from build123d import *

# Parameters (mm, degrees)
F0_R      = 15
F2_R      = 12.5
F4_R      = 10
F6_R      = 7.5
F8_R      = 5
F10_W     = 35
F10_H     = 35
F11_DEPTH = 1


with BuildPart() as f9:
    # F0 (on Top) → F9 section 0
    with BuildSketch(Plane.XY):
        Circle(F0_R)
    # F2 (on offset) → F9 section 1
    with BuildSketch(Plane.XY.offset(10)):
        Circle(F2_R)
    # F4 (on offset) → F9 section 2
    with BuildSketch(Plane.XY.offset(20)):
        Circle(F4_R)
    # F6 (on offset) → F9 section 3
    with BuildSketch(Plane.XY.offset(30)):
        Circle(F6_R)
    # F8 (on offset) → F9 section 4
    with BuildSketch(Plane.XY.offset(40)):
        Circle(F8_R)
    loft()

    # F10 (on Top) → F11 (join)
    with BuildSketch(Plane.XY):
        Rectangle(F10_W, F10_H)
    extrude(amount=-F11_DEPTH)


solid = f9.part
Verification items for the finished model (mm, model axes). A direction names the side the tool comes from. Give positions to 0.01 mm unless a question says otherwise; leave off trailing zeros. Answer as CSV lines item,"result". Start each with the question number.
1. Depth check by flat-ended pin: pin 1 (8 mm diameter, centred on x = -12.5, z = 9, fed in from -Y); pin 2 (5 mm diameter, centred on x = 12.5, z = 5.5, fed in from +Y); pin 3 (6 mm diameter, centred on x = 7.5, z = 7, fed in from -Y); pin 4 (1.5 mm diameter, centred on x = 9, z = 27.5, fed in from +Y). Enter the tip coordinate at first touch or a pass-through.
2. Thickness scan on line 1 (Z direction, x = 15, y = -5); line 2 (X direction, y = 10.5, z = 5.5); line 3 (Y direction, x = -9, z = 18). Record the ranges inside material, lowest first.
3. Set-up check for faces 1 (the face through (-13, -9, 0)), 2 (the face through (-0.2, -17.5, -0.5)): record each of +Z, -Z, +X, -X, +Y, -Y from which the full face is reachable in a straight line by a thin tool's end or side.
Derived:
1,pin 1,"y = -9.75"
1,pin 2,"y = 9.41"
1,pin 3,"y = -12.72"
1,pin 4,"through"
2,line 1,"-1 to 0"
2,line 2,"-8.68 to 8.68"
2,line 3,"-5.41 to 5.41"
3,face 1,"+Z"
3,face 2,"+Z, -Z, +X, -X, -Y"
